from build123d import *

# Parameters (mm, degrees)
SKETCH1_W           = 42
SKETCH1_H           = 15
BOSS_EXTRUDE1_DEPTH = 5
SKETCH2_R           = 1.115
CUT_EXTRUDE1_DEPTH  = 6
SKETCH3_W           = 15
SKETCH3_H           = 75.5
BOSS_EXTRUDE2_DEPTH = 5
SKETCH4_W           = 35
SKETCH4_H           = 10
BOSS_EXTRUDE3_DEPTH = 5
SKETCH5_W           = 10
SKETCH5_H           = 10
BOSS_EXTRUDE4_DEPTH = 5
SKETCH6_R           = 1.75
CUT_EXTRUDE2_DEPTH  = 6
SKETCH7_W           = 15
SKETCH7_H           = 0.2
CUT_EXTRUDE3_DEPTH  = 6
SKETCH8_W           = 2
SKETCH8_H           = 100.3
BOSS_EXTRUDE5_DEPTH = 10
CUT_EXTRUDE4_DEPTH  = 23


with BuildPart() as part:
    # Sketch1 → Boss-Extrude1 (new body)
    with BuildSketch(Plane(origin=(0, 0, 0), x_dir=(1, 0, 0), z_dir=(0, 1, 0))):
        with Locations((21, 7.5)):
            Rectangle(SKETCH1_W, SKETCH1_H)
    extrude(amount=BOSS_EXTRUDE1_DEPTH)

    # Sketch2 → Cut-Extrude1 (cut, through all)
    with BuildSketch(Plane(origin=(0, 5, 0), x_dir=(1, 0, 0), z_dir=(0, 1, 0))):
        with Locations((3, 7.5)):
            Circle(SKETCH2_R)
        with Locations((39, 7.5)):
            Circle(SKETCH2_R)
    extrude(amount=-CUT_EXTRUDE1_DEPTH, mode=Mode.SUBTRACT)

    # Sketch3 → Boss-Extrude2 (add)
    with BuildSketch(Plane(origin=(0, 5, 0), x_dir=(1, 0, 0), z_dir=(0, 1, 0))):
        with Locations((21, -37.75)):
            Rectangle(SKETCH3_W, SKETCH3_H)
    extrude(amount=-BOSS_EXTRUDE2_DEPTH)

    # Sketch4 → Boss-Extrude3 (add)
    with BuildSketch(Plane(origin=(0, 5, 0), x_dir=(1, 0, 0), z_dir=(0, 1, 0))):
        with Locations((21, -80.5)):
            Rectangle(SKETCH4_W, SKETCH4_H)
    extrude(amount=-BOSS_EXTRUDE3_DEPTH)

    # Sketch5 → Boss-Extrude4 (add)
    with BuildSketch(Plane(origin=(0, 5, 0), x_dir=(1, 0, 0), z_dir=(0, 1, 0))):
        with Locations((8.5, -90.5)):
            Rectangle(SKETCH5_W, SKETCH5_H)
        with Locations((33.5, -90.5)):
            Rectangle(SKETCH5_W, SKETCH5_H)
    extrude(amount=-BOSS_EXTRUDE4_DEPTH)

    # Sketch6 → Cut-Extrude2 (cut, through all)
    with BuildSketch(Plane(origin=(0, 5, 0), x_dir=(1, 0, 0), z_dir=(0, 1, 0))):
        with Locations((8.5, -90.5)):
            Circle(SKETCH6_R)
        with Locations((33.5, -90.5)):
            Circle(SKETCH6_R)
    extrude(amount=-CUT_EXTRUDE2_DEPTH, mode=Mode.SUBTRACT)

    # Sketch7 → Cut-Extrude3 (cut, through all)
    with BuildSketch(Plane(origin=(0, 5, 0), x_dir=(1, 0, 0), z_dir=(0, 1, 0))):
        with Locations((21, -85.4)):
            Rectangle(SKETCH7_W, SKETCH7_H)
    extrude(amount=-CUT_EXTRUDE3_DEPTH, mode=Mode.SUBTRACT)

    # Sketch8 → Boss-Extrude5 (add)
    with BuildSketch(Plane(origin=(0, 5, 0), x_dir=(1, 0, 0), z_dir=(0, 1, 0))):
        with Locations((21, -35.15)):
            Rectangle(SKETCH8_W, SKETCH8_H)
    extrude(amount=BOSS_EXTRUDE5_DEPTH)

    # Sketch9 → Cut-Extrude4 (cut, through all)
    with BuildSketch(Plane.ZY.offset(-20)):
        Polygon((-15, 15), (85.5, 5), (85.3, 15), align=None)
    extrude(amount=-CUT_EXTRUDE4_DEPTH, mode=Mode.SUBTRACT)


solid = part.part
Could you check a few things on this model? Use its own coordinates, in mm. A direction names the side the tool comes from. Coordinates: 2 decimals unless noted, no trailing zeros. Loops run counter-clockwise (first coordinate to the right, second up) from the corner with the lowest first, then second, coordinate; pieces in that order, holes last.
1. Imagine slicing it at B-B (y = 4). Please give me the cut outline in (x, z) (3 decimals).
2. We'd pull the mould along X, two halves only. Please class faces 1 (the face through (3.5, 3, 86)), 2 (the face through (42, 2, -7)), 3 (the face through (33, 3, 95.5)), 4 (the face through (9.4, 2.5, 89)): released by +X, released by -X, zero draft, split by the parting line, or undercut.
3. Imagine slicing it at A-A (x = 8.5). Please give me the cut outline in (y, z).
4. For P1, Ø4, axis at x = 18.5, y = 3, coming from the +Z side; P2, Ø5.5, axis at y = 3.5, z = 89, coming from the +X side; P3, Ø8, axis at y = 1.5, z = 55, coming from the +X side; P4, Ø2, axis at x = 11.5, z = 59.5, coming from the +Y side, each with a flat end and sliding along its axis, tell me the tip position at first contact or that it passes through.
5. Imagine slicing it at C-C (z = 15). Please give me the cut outline in (x, y).
6. For faces 5 (the face through (27, 5, 39)), 6 (the face through (14, 5, 39)), 7 (the face through (21, 4, -15)), 8 (the face through (35, 2, 0)), 9 (the face through (13.5, 3, 90)), which set-ups out of +Z, -Z, +X, -X, +Y, -Y let a thin tool reach every point of the face, with its end or its side?
7. I need wall thicknesses on L1, parallel to X at y = 3.7, z = -7.5 (3 decimals); L2, parallel to Z at x = 8.5, y = 3.3; L3, parallel to Z at x = 6, y = 1.25. Which ranges of each line are inside material? Lowest first, please.
8. Imagine slicing it at D-D (y = 12). Please give me the cut outline in (x, z).
Computed values:
1. outline: (0, -15) - (42, -15) - (42, 0) - (28.5, 0) - (28.5, 75.5) - (38.5, 75.5) - (38.5, 95.5) - (28.5, 95.5) - (28.5, 85.3) - (13.5, 85.3) - (13.5, 95.5) - (3.5, 95.5) - (3.5, 75.5) - (13.5, 75.5) - (13.5, 0) - (0, 0) - close; hole circle Ø2.23 at (3, -7.5); hole circle Ø3.5 at (8.5, 90.5); hole circle Ø3.5 at (33.5, 90.5); hole circle Ø2.23 at (39, -7.5)
2. face 1: released by -X
2. face 2: released by +X
2. face 3: zero draft
2. face 4: undercut
3. outline: (0, -15) - (5, -15) - (5, 0) - (0, 0) - close; (0, 75.5) - (5, 75.5) - (5, 88.75) - (0, 88.75) - close; (0, 92.25) - (5, 92.25) - (5, 95.5) - (0, 95.5) - close
4. P1: stops at z = 85.3
4. P2: stops at x = 38.5
4. P3: stops at x = 28.5
4. P4: passes through
5. outline: (13.5, 0) - (28.5, 0) - (28.5, 5) - (22, 5) - (22, 12.01) - (20, 12.01) - (20, 5) - (13.5, 5) - close
6. face 5: +Z, -Z, +X, +Y
6. face 6: +Z, -Z, -X, +Y
6. face 7: -Z, +X, -X, +Y, -Y
6. face 8: +X, +Y, -Y
6. face 9: +Z, +Y, -Y
7. L1: x = 0 to 1.885, 4.115 to 37.885, 40.115 to 42
7. L2: z = -15 to 0, 75.5 to 88.75, 92.25 to 95.5
7. L3: z = -15 to 0, 75.5 to 95.5
8. outline: (20, -15) - (22, -15) - (22, 15.15) - (20, 15.15) - close
